Part model, mm, in its own coordinate system. A direction names the side the tool comes from. Round coordinates to 2 decimals unless told otherwise and drop trailing zeros. Write each loop counter-clockwise with the first axis right and the second up, starting at its lowest first coordinate (ties: lowest second). Pieces come first, ordered by that corner, then holes. Notation, with made-up numbers: M 77.25,16.5 L 123.25,16.5 A15 ccw 123.25,39.5 Z; hole C 22,84 d11. An arc over 180 degrees is marked long. Use one line per item in the form item = value. Start each with the question number.
Item 1: Cut at A-A, the plane x = -57.5. Give the cut face in (y, z), then the cut area to 3 significant figures.
Item 2: Probe L1, parallel to Y at x = -50, z = 8.75; L2, parallel to Y at x = -70, z = 3; L3, parallel to Y at x = 21.5, z = 1.75. List the from-to ranges inside material, lowest first.
Item 3: Flat gauge pins, fed straight in: pin 1 Ø3 at (x, z) = (21, 3) entering from +Y; pin 2 Ø2 at (x, z) = (38.5, 3) entering from -Y; pin 3 Ø3 at (y, z) = (-8, 3) entering from -X. Where does each tip first touch, or does it go through?
Item 4: Cut at B-B, the plane y = 24. Give the cut face in (x, z).
Item 5: Cut at D-D, the plane y = -33.5. Give the cut face in (x, z).
Item 6: Cut at C-C, the plane z = 3.75. Give the cut face in (x, y), then the cut area to 3 significant figures.
Item 7: Mould opens along Y. For faces 1 (the face through (-74.54, 44.92, 4.93)), 2 (the face through (24.298, 38.128, 4.93)), 3 (the face through (-74.3, -45.5, 4.9)), 4 (the face through (-78.244, -25, 5)) say: +Y half, -Y half, draft (parallel to the pull), parting line (faces both ways), or undercut.
Item 8: Which spindle directions (+Z, -Z, +X, -X, +Y, -Y) get a long thin tool onto all of the face, cutting with end or side? Do faces 5 (the face through (-62, -15, 5)), 6 (the face through (-24.17, 25.78, 4.93)), 7 (the face through (-78.244, 26, 5)). Say none if no direction does.
Autodesk Inventor part; units mm, degrees
ref_plane "YZ Plane" through (0, 0, 0) normal (1, 0, 0) x (0, 1, 0)
ref_plane "XZ Plane" through (0, 0, 0) normal (0, 1, 0) x (-1, 0, 0)
ref_plane "XY Plane" through (0, 0, 0) normal (0, 0, 1) x (1, 0, 0)
sketch "스케치1" plane through (0, 0, 0) normal (0, 0, 1) x (1, 0, 0)
  line L0 (-26.6915, 0) -> (30.6457, 0)
  line L1 (0.0002, 26.0752) -> (0.0002, -24.1528)
  line L2 (-65.2443, -49.1703) -> (0.0002, -49.1703)
  line L3 (0.0002, 48.8297) -> (-65.2443, 48.8297)
  line L4 (-78.2443, -49.1703) -> (77.7557, 48.8632) construction
  line L5 (78.0463, -48.7061) -> (-78.2443, 48.8297) construction
  line L6 (-65.2443, 35.8297) -> (18.7557, 35.8297)
  line L7 (18.7557, 35.8297) -> (18.7557, -36.1703)
  line L8 (18.7557, -36.1703) -> (-65.2443, -36.1703)
  line L9 (-65.2443, -36.1703) -> (-65.2443, 35.8297)
  line L10 (56.7557, 17.5022) -> (56.7557, -17.4978)
  circle A0 centre (18.7557, 35.8297) radius 6
  circle A1 centre (-65.2443, 35.8297) radius 6
  circle A2 centre (18.7557, -36.1703) radius 6
  circle A3 centre (-65.2443, -36.1703) radius 6
  arc A4 (-65.2443, 48.8297) -> (-78.2443, 35.8297) centre (-65.2443, 35.8297) ccw
  arc A5 (-78.2443, -36.1703) -> (-65.2443, -49.1703) centre (-65.2443, -36.1703) ccw
  line L11 (77.7557, -19) -> (77.7557, 19)
  line L12 (0.0002, 48.8297) -> (82.2012, 48.8297) construction
  line L13 (-78.2443, -49.1703) -> (82.2012, -49.1703) construction
  line L14 (0.0002, -49.1703) -> (19.6899, -49.1703)
  line L15 (0.0002, 48.8297) -> (19.0402, 48.8297)
  line L16 (19.6899, -49.1703) -> (57.7958, -38.9598)
  line L17 (19.6899, -49.1703) -> (59.1401, -49.1703) construction
  line L18 (19.0402, 48.8297) -> (59.7283, 48.8297) construction
  line L19 (57.7958, -38.9598) -> (87.4943, -38.9598) construction
  line L20 (19.0402, 48.8297) -> (61.8181, 48.8297) construction
  line L21 (19.0402, 48.8297) -> (57.0006, 38.6583)
  line L22 (19.0402, 48.8297) -> (58.3397, 48.8297) construction
  line L23 (57.0006, 38.6583) -> (77.7557, 19)
  line L24 (57.7958, -38.9598) -> (77.7557, -19)
  arc A6 (10.0002, 19.0022) -> (-0.0006, 29.0001) centre (0.0002, 19.0001) ccw
  line L25 (-78.2443, 35.8297) -> (-78.2443, 15.0001)
  line L26 (-78.2443, -15.0002) -> (-78.2443, -36.1703)
  line L27 (10.0002, 19.0022) -> (55.2557, 19.0022)
  line L28 (55.2557, -18.9978) -> (9.1632, -18.9978)
  line L29 (-45.2992, -15.0002) -> (-78.2443, -15.0002)
  arc A7 (-45.2992, -15.0002) -> (-0.0006, -24.9934) centre (-9.1955, 40.9912) ccw
  arc A8 (-0.0006, 29.0001) -> (-45.2992, 15.0001) centre (-2.8258, -42.143) ccw
  arc A9 (-0.0006, -24.9934) -> (9.1632, -18.9978) centre (0.0002, -14.9938) ccw
  arc A10 (56.7557, 17.5022) -> (55.2557, 19.0022) centre (55.2557, 17.5022) ccw
  arc A11 (55.2557, -18.9978) -> (56.7557, -17.4978) centre (55.2557, -17.4978) ccw
  line L30 (-78.2443, 15.0001) -> (-45.2992, 15.0001)
  point P0 (0, 0)
  dimension "d0" = 156
  dimension "d1" = 98
  dimension "d2" = 13
  dimension "d4" = 13
  dimension "d5" = 84
  dimension "d6" = 38
  dimension "d8" = 12
  dimension "d9" = 12
  dimension "d10" = 12
  dimension "d11" = 12
  dimension "d12" = 13
  dimension "d15" = 38
  dimension "d17" = 15
  dimension "d21" = 15
  dimension "d23" = 45
  dimension "d27" = 20
  dimension "d29" = 3
  dimension "d30" = 3
  dimension "d31" = 30.0004
extrude "돌출1" add sketch "스케치1" along normal blind 10 contours A5 L26 L29 L9 A3 L8 A2 L7 L28 A11 L10 A10 L27 A0 L6 A1 L30 L25 A4 L3 L15 L21 L23 L11 L24 L16 L14 L2 | L29 A7 A9 L28 L7 A2 L8 A3 L9 | L9 A1 L6 A0 L7 L27 A6 A8 L30
properties part number "스케치02"
Model answer:
q1.outline = M -49.17,0 L -15,0 L -15,10 L -49.17,10 Z; M 15,0 L 48.83,0 L 48.83,10 L 15,10 Z
q1.area = 680 mm²
q2.L1 = -49.17 to -15, 15 to 48.83
q2.L2 = -48.27 to -39.83, -32.51 to -15, 15 to 32.17, 39.49 to 47.93
q2.L3 = -48.69 to -41.51, -30.83 to -19, 19 to 30.49, 41.17 to 48.17
q3.pin_1 = 48.71
q3.pin_2 = -44.4
q3.pin_3 = 56.76
q4.outline = M -78.24,0 L -29.18,0 L -29.18,10 L -78.24,10 Z; M 8.66,0 L 72.48,0 L 72.48,10 L 8.66,10 Z
q5.outline = M -78.24,0 L -70.62,0 L -70.62,10 L -78.24,10 Z; M -59.87,0 L 13.38,0 L 13.38,10 L -59.87,10 Z; M 24.13,0 L 63.26,0 L 63.26,10 L 24.13,10 Z
q6.outline = M -78.24,-36.17 A13 ccw -65.24,-49.17 L 19.69,-49.17 L 57.8,-38.96 L 77.76,-19 L 77.76,19 L 57,38.66 L 19.04,48.83 L -65.24,48.83 A13 ccw -78.24,35.83 L -78.24,15 L -45.3,15 A71.2 cw 0,29 A10 cw 10,19 L 55.26,19 A1.5 cw 56.76,17.5 L 56.76,-17.5 A1.5 cw 55.26,-19 L 9.16,-19 A10 cw 0,-24.99 A66.62 cw -45.3,-15 L -78.24,-15 Z; hole C -65.24,-36.17 d12; hole C -65.24,35.83 d12; hole C 18.76,-36.17 d12; hole C 18.76,35.83 d12
q6.area = 8,130 mm²
q7.face_1 = +Y half
q7.face_2 = undercut
q7.face_3 = -Y half
q7.face_4 = draft
q8.face_5 = +Z, -Z, -X
q8.face_6 = +Z, -Z
q8.face_7 = +Z, -Z, -X, +Y, -Y
